Input: part model. Units: mm. Frame: model coordinates. Face numbers are marked on the shaded views. A direction names the side the tool comes from. Round coordinates to 2 decimals unless told otherwise and drop trailing zeros. Loops run counter-clockwise (first coordinate to the right, second up) from the corner with the lowest first, then second, coordinate; pieces in that order, holes last. Notation, with made-up numbers: M -23,43.25 L -18,43.25 A29 ccw -18,79.25 Z; hole C 63,31.5 d6. An arc over 180 degrees is marked long. Put each result on its own line as item: value. Start each with the question number.
1) Reachability of the marked faces 1, 2, 3, 4 and 5 from +Z, -Z, +X, -X, +Y, -Y: full face, straight path, thin tool, end or side. Return the list, or none.
2) Section B-B on y = -14.25. Output: boundary loops of the cut face in (x, z), plus the area to 3 significant figures.
3) Line query: probe 1 along Y at (x, z) = (-0.5, -0.5); probe 2 along Z at (x, y) = (-12.72, -22.75); probe 3 along Y at (x, z) = (7, -8). Output: solid intervals per line, ascending.
4) Section C-C on y = -9. Output: boundary loops of the cut face in (x, z).
5) Pin query (flat end, axial travel): pin 1 (1.5 mm diameter, centred on x = -1.5, z = -0.5, fed in from +Y); pin 2 (1.5 mm diameter, centred on x = -14, z = 0.5, fed in from +Y); pin 3 (0.6 mm diameter, centred on x = 13.5, y = -23, fed in from +Z); pin 4 (1.3 mm diameter, centred on x = 2.93, z = -15.65, fed in from +Y). Return the tip coordinate at first contact, or that it passes through.
6) Section A-A on z = 0. Output: boundary loops of the cut face in (x, y).
Autodesk Inventor part; units mm, degrees
ref_plane "YZ Plane" through (0, 0, 0) normal (1, 0, 0) x (0, 1, 0)
ref_plane "XZ Plane" through (0, 0, 0) normal (0, 1, 0) x (-1, 0, 0)
ref_plane "XY Plane" through (0, 0, 0) normal (0, 0, 1) x (1, 0, 0)
sketch "Sketch1" plane through (0, 0, 0) normal (0, 0, 1) x (1, 0, 0)
  line L0 (2.9264, -5.1404) -> (5.6442, -5.1404)
  line L1 (5.6442, -5.1404) -> (5.6442, -6.4866)
  line L2 (5.6442, -6.4866) -> (6.9015, -6.4866)
  line L3 (6.9015, -6.4866) -> (6.9015, -11.2364)
  line L4 (6.9015, -11.2364) -> (12.0958, -11.2364)
  line L5 (12.0958, -11.2364) -> (16.744, -13.1668)
  line L6 (16.744, -13.1668) -> (16.744, -22.006)
  line L7 (16.744, -22.006) -> (2.9264, -22.006)
  line L8 (2.9264, -22.006) -> (2.9264, -5.1404)
  point P0 (0, 0)
  dimension "d0" = 10.7696
  dimension "d1" = 8.8392
  dimension "d2" = 4.6482
  dimension "d3" = 13.8176
  dimension "d4" = 16.8656
  dimension "d5" = 1.3462
  dimension "d6" = 2.7178
  dimension "d7" = 3.9751
revolve "Revolution1" add sketch "Sketch1" angle 360 about axis through (2.9264, -22.006, 0) along (0, 1, 0)
sketch "Sketch2" plane through (2.9264, -22.006, 0) normal (0, -1, 0) x (1, 0, 0)
  circle A0 centre (0, 0) radius 13.8176
  line L0 (6.1468, 2.9718) -> (15.6464, 2.9718)
  line L1 (18.6182, 0) -> (18.6182, 0)
  line L2 (15.6464, -2.9718) -> (6.1468, -2.9718)
  line L3 (2.9718, 6.1468) -> (2.9718, 15.6464)
  line L4 (0, 18.6182) -> (0, 18.6182)
  line L5 (-2.9718, 15.6464) -> (-2.9718, 6.1468)
  line L6 (-6.1468, 2.9718) -> (-15.6464, 2.9718)
  line L7 (-18.6182, 0) -> (-18.6182, 0)
  line L8 (-15.6464, -2.9718) -> (-6.1468, -2.9718)
  line L9 (-2.9718, -6.1468) -> (-2.9718, -15.6464)
  line L10 (0, -18.6182) -> (0, -18.6182)
  line L11 (2.9718, -15.6464) -> (2.9718, -6.1468)
  arc A1 (-6.1468, 2.9718) -> (-2.9718, 6.1468) centre (-6.1468, 6.1468) ccw
  arc A2 (2.9718, 6.1468) -> (6.1468, 2.9718) centre (6.1468, 6.1468) ccw
  arc A3 (6.1468, -2.9718) -> (2.9718, -6.1468) centre (6.1468, -6.1468) ccw
  arc A4 (-2.9718, -6.1468) -> (-6.1468, -2.9718) centre (-6.1468, -6.1468) ccw
  arc A5 (18.6182, 0) -> (15.6464, 2.9718) centre (15.6464, 0) ccw
  arc A6 (15.6464, -2.9718) -> (18.6182, 0) centre (15.6464, 0) ccw
  arc A7 (2.9718, 15.6464) -> (0, 18.6182) centre (0, 15.6464) ccw
  arc A8 (0, 18.6182) -> (-2.9718, 15.6464) centre (0, 15.6464) ccw
  arc A9 (-15.6464, 2.9718) -> (-18.6182, 0) centre (-15.6464, 0) ccw
  arc A10 (-18.6182, 0) -> (-15.6464, -2.9718) centre (-15.6464, 0) ccw
  arc A11 (-2.9718, -15.6464) -> (0, -18.6182) centre (0, -15.6464) ccw
  arc A12 (0, -18.6182) -> (2.9718, -15.6464) centre (0, -15.6464) ccw
  circle A13 centre (0, 15.6464) radius 1.0668
  circle A14 centre (15.6464, 0) radius 1.0668
  circle A15 centre (-15.6464, 0) radius 1.0668
  circle A16 centre (0, -15.6464) radius 1.0668
  point P0 (-2.9264, 0)
  dimension "d9" = 3.175
  dimension "d10" = 5.9436
  dimension "d11" = 2.9718
  dimension "d12" = 5.9436
  dimension "d13" = 15.6464
  dimension "d14" = 15.6464
  dimension "d15" = 15.6464
  dimension "d16" = 2.1336
extrude "Extrusion1" add sketch "Sketch2" along normal blind 1.1684 contours A0 L2 A3 L11 L9 A4 L8 L6 A1 L5 L3 A2 L0 | A0 L0 A5 A6 L2 | A0 L5 A8 A7 L3 | L11 A12 A11 L9 A0 | A0 L8 A10 A9 L6
equation "\"d12\" = d10"
equation "\"d14\" = d13"
equation "\"d15\" = d13"
properties part number "Lift_Motor"
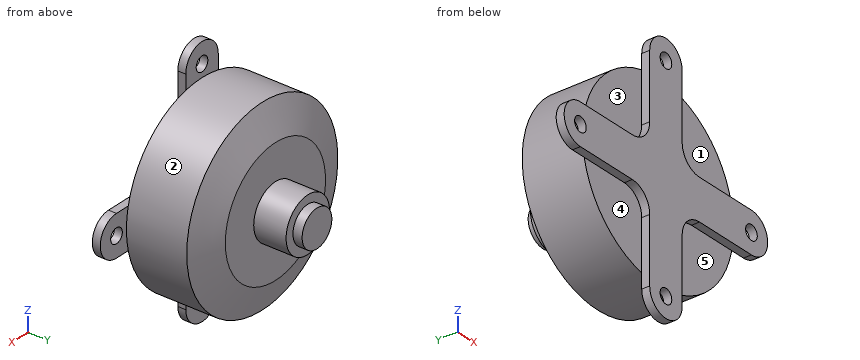
Geometry results:
1. face 1: +Z, +X, -Y
1. face 2: +Y
1. face 3: +Z, -X, -Y
1. face 4: -Z, -X, -Y
1. face 5: -Z, +X, -Y
2. outline: C 2.93,0 d27.64
2. area: 600 mm²
3. probe 1: y = -23.17 to -6.49
3. probe 2: z = -2.97 to -1.07, 1.07 to 2.97
3. probe 3: y = -22.01 to -11.24
4. outline: C 2.93,0 d7.95
5. pin 1: stops at y = -6.49
5. pin 2: stops at y = -22.01
5. pin 3: stops at z = 2.97
5. pin 4: passes through
6. outline: M -15.69,-23.17 L -13.79,-23.17 L -13.79,-22.01 L -15.69,-22.01 Z; M -11.65,-23.17 L 17.51,-23.17 L 17.51,-22.01 L 16.74,-22.01 L 16.74,-13.17 L 12.1,-11.24 L 6.9,-11.24 L 6.9,-6.49 L 5.64,-6.49 L 5.64,-5.14 L 0.21,-5.14 L 0.21,-6.49 L -1.05,-6.49 L -1.05,-11.24 L -6.24,-11.24 L -10.89,-13.17 L -10.89,-22.01 L -11.65,-22.01 Z; M 19.64,-23.17 L 21.54,-23.17 L 21.54,-22.01 L 19.64,-22.01 Z
